```python
from build123d import *

# Parameters (mm, degrees)
BOSS_EXTRUDE1_DEPTH = 6.35
SKETCH2_W           = 177.8
SKETCH2_H           = 215.9
CUT_EXTRUDE2_DEPTH  = 6.35


with BuildPart() as part:
    # Sketch1 → Boss-Extrude1 (new body)
    with BuildSketch(Plane(origin=(0, 0, 0), x_dir=(1, 0, 0), z_dir=(0, 1, 0))):
        Polygon((-65.292450766, -101.6), (-39.892450766, -101.6), (-39.892450766, -107.95), (-14.492450766, -107.95), (-14.492450766, -101.6), (10.907549234, -101.6), (10.907549234, -107.95), (36.307549234, -107.95), (36.307549234, -101.6), (61.707549234, -101.6), (61.707549234, -107.95), (87.107549234, -107.95), (87.107549234, -101.6), (112.507549234, -101.6), (112.507549234, -107.95), (137.907549234, -107.95), (137.907549234, -101.6), (163.307549234, -101.6), (163.307549234, -107.95), (188.707549234, -107.95), (188.707549234, -101.6), (220.457549234, -101.6), (220.457549234, -76.2), (214.107549234, -76.2), (214.107549234, -50.8), (220.457549234, -50.8), (220.457549234, -25.4), (214.107549234, -25.4), (214.107549234, 0), (220.457549234, 0), (220.457549234, 25.4), (214.107549234, 25.4), (214.107549234, 50.8), (220.457549234, 50.8), (220.457549234, 76.2), (214.107549234, 76.2), (214.107549234, 101.6), (220.457549234, 101.6), (220.457549234, 127), (214.107549234, 127), (214.107549234, 152.4), (220.457549234, 152.4), (220.457549234, 177.8), (214.107549234, 177.8), (214.107549234, 209.55), (188.707549234, 209.55), (188.707549234, 203.2), (163.307549234, 203.2), (163.307549234, 209.55), (137.907549234, 209.55), (137.907549234, 203.2), (112.507549234, 203.2), (112.507549234, 209.55), (87.107549234, 209.55), (87.107549234, 203.2), (61.707549234, 203.2), (61.707549234, 209.55), (36.307549234, 209.55), (36.307549234, 203.2), (10.907549234, 203.2), (10.907549234, 209.55), (-14.492450766, 209.55), (-14.492450766, 203.2), (-39.892450766, 203.2), (-39.892450766, 209.55), (-65.292450766, 209.55), (-65.292450766, 203.2), (-97.042450766, 203.2), (-97.042450766, 177.8), (-90.692450766, 177.8), (-90.692450766, 152.4), (-97.042450766, 152.4), (-97.042450766, 127), (-90.692450766, 127), (-90.692450766, 101.6), (-97.042450766, 101.6), (-97.042450766, 76.2), (-90.692450766, 76.2), (-90.692450766, 50.8), (-97.042450766, 50.8), (-97.042450766, 25.4), (-90.692450766, 25.4), (-90.692450766, 0), (-97.042450766, 0), (-97.042450766, -25.4), (-90.692450766, -25.4), (-90.692450766, -50.8), (-97.042450766, -50.8), (-97.042450766, -76.2), (-90.692450766, -76.2), (-90.692450766, -107.95), (-65.292450766, -107.95), align=None)
    extrude(amount=BOSS_EXTRUDE1_DEPTH)

    # Sketch2 → Cut-Extrude2 (cut)
    with BuildSketch(Plane(origin=(0, 6.35, 0), x_dir=(1, 0, 0), z_dir=(0, 1, 0))):
        with Locations((61.707549234, 50.8)):
            Rectangle(SKETCH2_W, SKETCH2_H)
    extrude(amount=-CUT_EXTRUDE2_DEPTH, mode=Mode.SUBTRACT)


solid = part.part
```
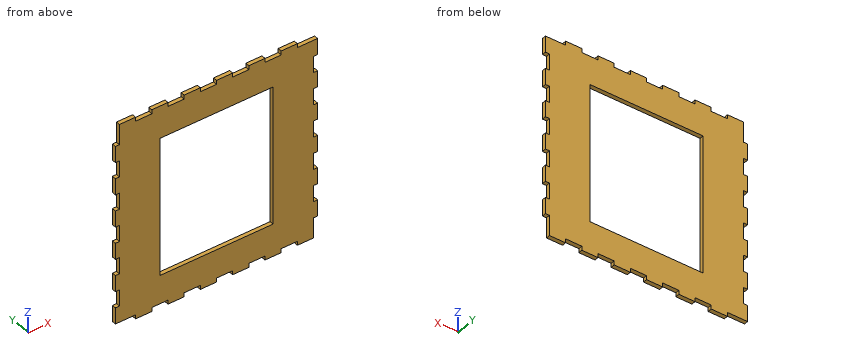
CAD build for the part. Positions are in the model's coordinates, mm. Coordinates: 2 decimals unless noted, no trailing zeros. Write each loop counter-clockwise with the first axis right and the second up, starting at its lowest first coordinate (ties: lowest second). Pieces come first, ordered by that corner, then holes. Notation, with made-up numbers: (-12, 53.5) -> (36, 53.5) arc R16 ccw to (36, 58.5) -> close; hole circle Ø5 at (22.25, -21). An arc over 180 degrees is marked (long way). Return JSON: item names as keys, results as strings. Group by question number.
Q1. Cut at C-C, the plane z = -190. Give the cut face in (x, y), then the cut area to 3 significant figures.
Q2. Cut at D-D, the plane x = -45.5. Give the cut face in (y, z), then the cut area to 3 significant figures.
Q3. Cut at A-A, the plane x = 94.5. Give the cut face in (y, z).
Q4. Drill centre lines: line 1 (X direction, y = 3, z = -96); line 2 (X direction, y = 2, z = -22.5); line 3 (Z direction, x = 16, y = 3.5). Where is each one in solid material? Low to high.
Q5. Flat gauge pins, fed straight in: pin 1 (3 mm diameter, centred on y = 3, z = -92.5, fed in from +X); pin 2 (3 mm diameter, centred on x = -47.5, y = 4.5, fed in from +Z); pin 3 (3 mm diameter, centred on y = 3.5, z = 106, fed in from +X); pin 4 (10 mm diameter, centred on x = -47, z = 14.5, fed in from -Y). Where does each tip first touch, or does it go through?
Q6. Cut at B-B, the plane z = -107. Give the cut face in (x, y), then the cut area to 3 significant figures.
Returned:
{
 "1": {"outline": "(-97.04, 0) -> (214.11, 0) -> (214.11, 6.35) -> (-97.04, 6.35) -> close", "area": "1,980 mm2"},
 "2": {"outline": "(0, -209.55) -> (6.35, -209.55) -> (6.35, 101.6) -> (0, 101.6) -> close", "area": "1,980 mm2"},
 "3": {"outline": "(0, -209.55) -> (6.35, -209.55) -> (6.35, -158.75) -> (0, -158.75) -> close; (0, 57.15) -> (6.35, 57.15) -> (6.35, 101.6) -> (0, 101.6) -> close"},
 "4": {"line 1": "x = -97.04 to -27.19, 150.61 to 214.11", "line 2": "x = -90.69 to -27.19, 150.61 to 220.46", "line 3": "z = -203.2 to -158.75, 57.15 to 107.95"},
 "5": {"pin 1": "stops at x = 214.11", "pin 2": "stops at z = 101.6", "pin 3": "stops at x = 188.71", "pin 4": "stops at y = 0"},
 "6": {"outline": "(-90.69, 0) -> (-27.19, 0) -> (-27.19, 6.35) -> (-90.69, 6.35) -> close; (150.61, 0) -> (220.46, 0) -> (220.46, 6.35) -> (150.61, 6.35) -> close", "area": "847 mm2"}
}
